Check sheet for the modelled part. Datum: model origin and axes. Units: mm. Face numbers are marked on the shaded views. A direction names the side the tool comes from. Give positions to 0.01 mm unless a question says otherwise; leave off trailing zeros. Order: outer loops, then holes, each group sorted by start corner. A loop starts at its lowest first (then second) coordinate and runs counter-clockwise, first axis right, second up. Notation, with made-up numbers: (-13, -16) -> (38, -16) arc R31 ccw to (38, 11) -> close; hole circle Ø5 at (6, 17). An arc over 180 degrees is marked (long way). Answer in a Markdown table with one row per item. Add a question column.
(1) Set-up check for the marked faces 1 and 2: record each of +Z, -Z, +X, -X, +Y, -Y from which the full face is reachable in a straight line by a thin tool's end or side.
(2) Cross-section at C-C (x = 7.5). Record the cut outline in (y, z).
(3) Release check for a two-part mould opening along X. For the marked faces 3, 4 and 5 record: released by +X, released by -X, zero draft, split by the parting line, or undercut.
(4) Cross-section at B-B (y = 1). Record the cut outline in (x, z).
(5) Go/stop test with flat-tipped pins: pin 1 (4 mm diameter, centred on y = 38, z = 22.5, fed in from +X); pin 2 (15.5 mm diameter, centred on x = 0, z = 15, fed in from -Y); pin 3 (8 mm diameter, centred on x = -9.5, z = 4.5, fed in from +Y). Record where each tip stops, or that it passes through.
(6) Cross-section at D-D (y = 28.5). Record the cut outline in (x, z).
(7) Cross-section at A-A (z = 15). Record the cut outline in (x, y), then the cut area to 3 significant figures.
(8) Thickness scan on L1, parallel to X at y = 28, z = 6; L2, parallel to Z at x = 0, y = -10.25; L3, parallel to Y at x = 0.5, z = 24. Record the ranges inside material, lowest first. Write a range as [from, to].
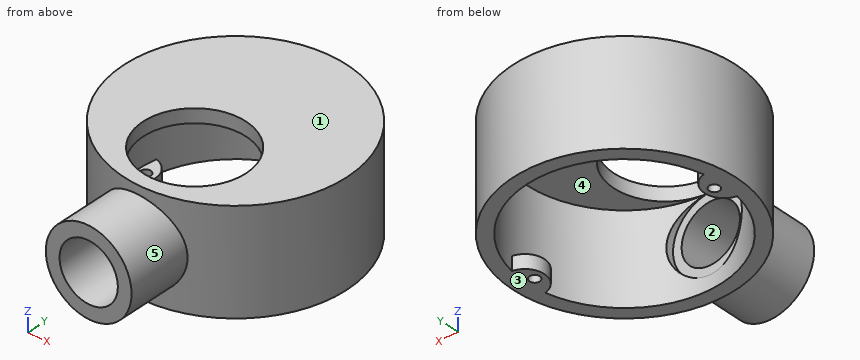
```python
from build123d import *

# Parameters (mm, degrees)
F0_R      = 12.5
F1_DEPTH  = 20
F2_R      = 32.5
F3_DEPTH  = 30
F4_R      = 28.5
F5_DEPTH  = 26
F6_R      = 11
F7_DEPTH  = 19.5
F8_R      = 15
F9_DEPTH  = 44.3
F10_R     = 8.5
F11_DEPTH = 41.2
F12_R     = 1.5
F13_DEPTH = 4


with BuildPart() as f1:
    # F0 (on Front) → F1 (new body, symmetric)
    with BuildSketch(Plane.XZ):
        with Locations((0, 15)):
            Circle(F0_R)
    extrude(amount=F1_DEPTH, both=True)

    # F2 (on Top) → F3 (join)
    with BuildSketch(Plane.XY):
        with Locations((0, 28.5)):
            Circle(F2_R)
    extrude(amount=F3_DEPTH)

    # F4 (on Top) → F5 (cut)
    with BuildSketch(Plane.XY):
        with Locations((0, 28.5)):
            Circle(F4_R)
    extrude(amount=F5_DEPTH, mode=Mode.SUBTRACT)

    # F6 (on Front) → F7 (cut)
    with BuildSketch(Plane.XZ):
        with Locations((0, 15)):
            Circle(F6_R)
    extrude(amount=-F7_DEPTH, mode=Mode.SUBTRACT)

    # F8 (on Top) → F9 (cut)
    with BuildSketch(Plane.XY):
        with Locations((0, 15)):
            Circle(F8_R)
    extrude(amount=F9_DEPTH, mode=Mode.SUBTRACT)

    # F10 (on Front) → F11 (cut)
    with BuildSketch(Plane.XZ):
        with Locations((0, 15)):
            Circle(F10_R)
    extrude(amount=F11_DEPTH, mode=Mode.SUBTRACT)

    # F12 (on Top) → F13 (join)
    with BuildSketch(Plane.XY):
        with BuildLine():
            Line((29, 28.5), (29, 34.138157))
            ThreePointArc((29, 34.138157), (23.361843, 28.5), (29, 22.861843))
            Line((29, 22.861843), (29, 28.5))
        make_face()
        with Locations((26.180921, 28.5)):
            Circle(F12_R, mode=Mode.SUBTRACT)
        with BuildLine():
            ThreePointArc((-29, 22.861843), (-23.361843, 28.5), (-29, 34.138157))
            Line((-29, 34.138157), (-29, 28.5))
            Line((-29, 28.5), (-29, 22.861843))
        make_face()
        with Locations((-26.180921, 28.5)):
            Circle(F12_R, mode=Mode.SUBTRACT)
    extrude(amount=F13_DEPTH)


solid = f1.part
```
Answer below:
| question | item | result |
|---|---|---|
| 1 | face 1 | +Z, +X, -X, +Y, -Y |
| 1 | face 2 | -Y |
| 2 | outline | (-20, 5) -> (-3.12, 5) -> (-3.12, 0) -> (1, 0) -> (1, 6.95) -> (0, 6.95) -> (0, 11) -> (-20, 11) -> close; (-20, 19) -> (0, 19) -> (0, 23.05) -> (1, 23.05) -> (1, 26) -> (2.01, 26) -> (2.01, 30) -> (-3.12, 30) -> (-3.12, 25) -> (-20, 25) -> close; (27.99, 26) -> (56, 26) -> (56, 0) -> (60.12, 0) -> (60.12, 30) -> (27.99, 30) -> close |
| 3 | face 3 | zero draft |
| 3 | face 4 | undercut |
| 3 | face 5 | split by the parting line |
| 4 | outline | (-17.32, 0) -> (-7.48, 0) -> (-7.48, 6.94) arc R11 cw to (-7.48, 23.06) -> (-7.48, 26) -> (-5.39, 26) -> (-5.39, 30) -> (-17.32, 30) -> close; (5.39, 26) -> (7.48, 26) -> (7.48, 23.06) arc R11 cw to (7.48, 6.94) -> (7.48, 0) -> (17.32, 0) -> (17.32, 30) -> (5.39, 30) -> close |
| 5 | pin 1 | stops at x = 31.62 |
| 5 | pin 2 | stops at y = 55.93 |
| 5 | pin 3 | stops at y = 60.53 |
| 6 | outline | (-32.5, 0) -> (-27.68, 0) -> (-27.68, 4) -> (-28.5, 4) -> (-28.5, 26) -> (-6.54, 26) -> (-6.54, 30) -> (-32.5, 30) -> close; (-24.68, 0) -> (-23.36, 0) -> (-23.36, 4) -> (-24.68, 4) -> close; (6.54, 26) -> (28.5, 26) -> (28.5, 4) -> (27.68, 4) -> (27.68, 0) -> (32.5, 0) -> (32.5, 30) -> (6.54, 30) -> close; (23.36, 0) -> (24.68, 0) -> (24.68, 4) -> (23.36, 4) -> close |
| 7 | outline | (-12.5, -20) -> (-8.5, -20) -> (-8.5, 0) -> (-11, 0) -> (-11, 2.21) arc R28.5 cw (long way) to (11, 2.21) -> (11, 0) -> (8.5, 0) -> (8.5, -20) -> (12.5, -20) -> (12.5, -1.5) arc R32.5 ccw (long way) to (-12.5, -1.5) -> close |
| 7 | area | 831 mm² |
| 8 | L1 | x = [-32.5, -28.5], [28.5, 32.5] |
| 8 | L2 | z = [2.5, 6.5], [23.5, 27.5] |
| 8 | L3 | y = [-20, 0], [57, 61] |
